Check sheet for the drawn part. Datum: minimum x, y, z corner. Units: mm. Give positions to 0.01 mm unless a question says otherwise; leave off trailing zeros. Loops run counter-clockwise (first coordinate to the right, second up) from the corner with the lowest first, then second, coordinate; pieces in that order, holes last. Notation, with made-up numbers: M 61.5,13 L 100.5,13 A32 cw 100.5,51 Z; hole C 16.25,31 d11. An arc over 180 degrees is marked long. Write each question's results on one line, items separated by ' | '. Start each with the question number.
1. Go/stop test with a flat-tipped pin: pin 1 (2 mm diameter, centred on x = 22.5, z = 27.5, fed in from -Y). Record where the tip stops, or that it passes through.
2. Sectioned sample at A-A on x = 12.7. Record the cut outline in (y, z) (1 decimal), and give its area (3 significant figures).
3. Material ranges on line 1 along Y through (x, z) = (12.7, 18.5) (1 decimal); line 2 along Z through (x, y) = (12, 5.25); line 3 along Y through (x, z) = (10, 27) (1 decimal), recorded low to high.
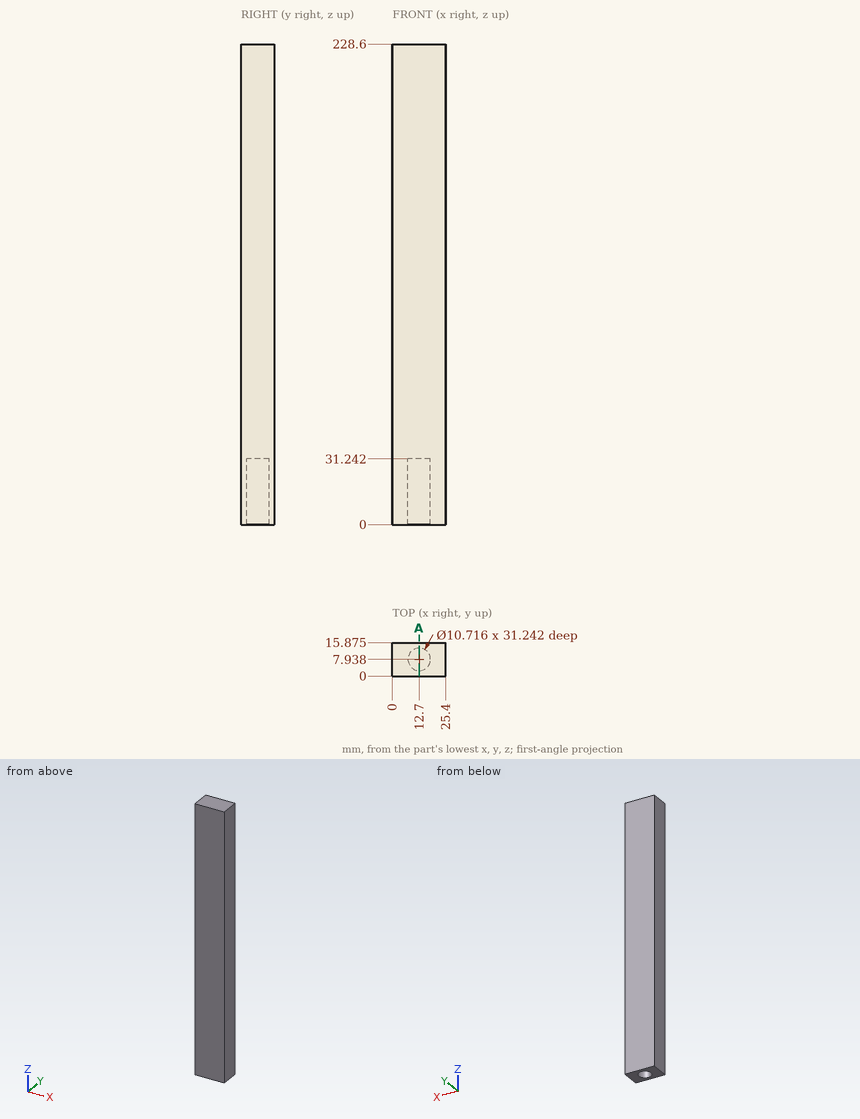
Output values:
1) pin 1: y = 0
2) outline: M 0,0 L 2.6,0 L 2.6,31.2 L 13.3,31.2 L 13.3,0 L 15.9,0 L 15.9,228.6 L 0,228.6 Z | area: 3,290 mm2
3) line 1: 0 to 2.6, 13.3 to 15.9 | line 2: 31.24 to 228.6 | line 3: 0 to 3.3, 12.6 to 15.9
